from build123d import *

# Parameters (mm, degrees)
CYLINDER010_R        = 31.25
CYLINDER010_DEPTH    = 71.327905
POCKET071_DEPTH      = 43.251
POCKET071_DEPTH_BACK = 28.078905
POCKET084_DEPTH      = 8.5
POCKET085_DEPTH      = 31.251
POCKET085_DEPTH_BACK = 31.251
GROOVE_ANGLE         = -90
POCKET192_DEPTH      = 220.995838
CHAMFER003_SIZE      = 0.4


with BuildPart() as part:
    # Cylinder010 → Cylinder010 (join)
    with BuildSketch(Plane.XY.offset(-43.25)):
        Circle(CYLINDER010_R)
    extrude(amount=CYLINDER010_DEPTH)

    # Sketch132 → Pocket071 (cut, two sides)
    with BuildSketch(Plane.XY) as pocket071_sk:
        with BuildLine():
            Line((-13.322913, 15.25), (13.322913, 15.25))
            ThreePointArc((15.25, 13.322913), (14.318912, 14.318912), (13.322913, 15.25))
            Line((15.25, 13.322913), (15.25, -13.322913))
            ThreePointArc((13.322913, -15.25), (14.318912, -14.318912), (15.25, -13.322913))
            Line((-13.322913, -15.25), (13.322913, -15.25))
            ThreePointArc((-15.25, -13.322913), (-14.318912, -14.318912), (-13.322913, -15.25))
            Line((-15.25, 13.322913), (-15.25, -13.322913))
            ThreePointArc((-13.322913, 15.25), (-14.318912, 14.318912), (-15.25, 13.322913))
        make_face()
    extrude(amount=-POCKET071_DEPTH, mode=Mode.SUBTRACT)
    extrude(pocket071_sk.sketch, amount=POCKET071_DEPTH_BACK, mode=Mode.SUBTRACT)

    # Sketch140 → Pocket084 (cut)
    with BuildSketch(Plane.XY.offset(28.077905)):
        with BuildLine():
            ThreePointArc((-13.322913, 15.25), (-20.25, 0), (-13.322913, -15.25))
            Line((-13.322913, 15.25), (-13.322913, -15.25))
        make_face()
    extrude(amount=-POCKET084_DEPTH, mode=Mode.SUBTRACT)

    # Sketch130 → Pocket085 (cut, two sides)
    with BuildSketch(Plane.XZ) as pocket085_sk:
        Polygon((-33.55, -33.55), (33.55, 33.55), (33.55, -61.55), (-33.55, -61.55), align=None)
        with BuildLine():
            ThreePointArc((2.2, 16), (0, 18.2), (-2.2, 16))
            Line((-2.2, 16), (-2.2, 12))
            ThreePointArc((-2.2, 12), (0, 9.8), (2.2, 12))
            Line((2.2, 16), (2.2, 12))
        make_face()
    extrude(amount=-POCKET085_DEPTH, mode=Mode.SUBTRACT)
    extrude(pocket085_sk.sketch, amount=POCKET085_DEPTH_BACK, mode=Mode.SUBTRACT)

    # Sketch → Groove (revolve, symmetric, cut)
    with BuildSketch(Plane.XZ) as groove_sk:
        Polygon((-20.25, 19.577905), (0, 19.577905), (0, -0.672095), align=None)
    revolve(axis=Axis((0, 0, 0), (0, 0, 1)), revolution_arc=GROOVE_ANGLE / 2, mode=Mode.SUBTRACT)
    revolve(groove_sk.sketch, axis=Axis((0, 0, 0), (0, 0, -1)), revolution_arc=GROOVE_ANGLE / 2, mode=Mode.SUBTRACT)

    # Sketch131 → Pocket192 (cut, through all)
    with BuildSketch(Plane.XZ.offset(19.5)):
        with BuildLine():
            ThreePointArc((4, 16), (0, 20), (-4, 16))
            Line((-4, 16), (-4, 12))
            ThreePointArc((-4, 12), (0, 8), (4, 12))
            Line((4, 16), (4, 12))
        make_face()
    pocket192 = extrude(amount=POCKET192_DEPTH, mode=Mode.SUBTRACT)

    # Mirrored009: Pocket192 across XZ
    add(pocket192.mirror(Plane.XZ), mode=Mode.SUBTRACT)

    # Chamfer003
    chamfer003_edges = [part.edges().sort_by_distance(p)[0] for p in [
        (-31.25, 0, 28.077905),
        (28.077905, 0, 28.077905),
        (14.318912, -14.318912, 28.077905),
        (15.25, 0, 28.077905),
        (14.318912, 14.318912, 28.077905),
        (0, 15.25, 28.077905),
        (-14.318912, 14.318912, 28.077905),
        (-20.25, 0, 28.077905),
        (-14.318912, -14.318912, 28.077905),
        (0, -15.25, 28.077905),
    ]]
    chamfer(chamfer003_edges, length=CHAMFER003_SIZE)


with BuildPart() as part_1:
    # Body022026 placement: moved
    add(part.part.moved(Location((-3.125, 0, 854.79899))))


solid = part_1.part
Work out the finished part from the listing and answer in its coordinate system (mm). A direction names the side the tool comes from. Coordinates: 2 decimals unless noted, no trailing zeros. Write each loop counter-clockwise with the first axis right and the second up, starting at its lowest first coordinate (ties: lowest second). Pieces come first, ordered by that corner, then holes.
1. Consider line 1 along Y through (x, z) = (-8, 869.5); line 2 along Y through (x, z) = (-14.5, 856); line 3 along X through (y, z) = (0, 866) (3 decimals). Determine where each line is inside the solid, lowest interval first.
Results list:
line 1: y = -30.87 to -15.25, 15.25 to 30.87
line 2: y = -29.11 to -15.25, 15.25 to 29.11
line 3: x = -34.375 to -18.375
2. The part is cut by section B-B, the plane z = 856.5. Write down the section's boundary in (x, y) (3 decimals).
Results list:
outline: (-18.375, -13.323) - (-18.375, 13.323) arc R20.25 cw to (-16.448, 15.25) - (-1.424, 15.25) - (-1.424, 31.204) arc R31.25 ccw (long way) to (-1.424, -31.204) - (-1.424, -15.25) - (-16.448, -15.25) arc R20.25 cw to start
3. For faces 1 (the cylindrical face through (-3.2, 17.3, 864.6)), 2 (the conical face through (-21, 0, 872)), 3 (the flat face through (0.875, 25, 869)), 4 (the cylindrical face through (11.18, -14.33, 875.4)), determine the directions among +Z, -Z, +X, -X, +Y, -Y from which every point of the face is accessible in a straight line to the end or side of a thin tool.
Results list:
face 1: +Y, -Y
face 2: +Z
face 3: +Y
face 4: +Z, -Z
4. For a pull along X with two mould halves and no side action, classify faces 5 (the conical face through (11.348, -14.443, 882.674)), 6 (the cylindrical face through (-34.353, 1.163, 859.148)) as +X half, -X half, draft (parallel to the pull), parting line (faces both ways), or undercut.
Results list:
face 5: undercut
face 6: parting line
5. Flat-ended cylindrical pins translate along their axes: pin 1 (3 mm diameter, centred on y = 18.5, z = 869, fed in from +X); pin 2 (6 mm diameter, centred on y = 4, z = 878, fed in from -X); pin 3 (2.5 mm diameter, centred on x = -5, z = 869.5, fed in from +Y); pin 4 (10 mm diameter, centred on x = -0.5, z = 853, fed in from +Y). Find the tip coordinate at first contact, or state that the pin passes through.
Results list:
pin 1: stops at x = 12.58
pin 2: stops at x = -34.36
pin 3: stops at y = 19.5
pin 4: stops at y = 31.25
6. The part is cut by section D-D, the plane z = 831. Write down the section's boundary in (x, y) (3 decimals).
Results list:
outline: (-26.924, -20.253) - (-26.924, 20.253) arc R31.25 ccw to start
7. The part is cut by section A-A, the plane y = 0. Write down the section's boundary in (x, z) (3 decimals).
Results list:
outline: (-34.375, 823.549) - (-18.375, 839.549) - (-18.375, 869.377) - (-23.375, 874.377) - (-23.375, 882.477) - (-23.775, 882.877) - (-33.975, 882.877) - (-34.375, 882.477) - close; (12.125, 870.049) - (24.67, 882.594) - (24.553, 882.877) - (12.525, 882.877) - (12.125, 882.477) - close
8. The part is cut by section C-C, the plane z = 844.5. Write down the section's boundary in (x, y) (3 decimals), and give its area (3 significant figures).
Results list:
outline: (-18.375, -13.323) - (-18.375, 13.323) arc R20.25 cw to (-16.448, 15.25) - (-13.424, 15.25) - (-13.424, 29.504) arc R31.25 ccw to (-13.424, -29.504) - (-13.424, -15.25) - (-16.448, -15.25) arc R20.25 cw to start
area: 755 mm2
